For this review, take the finished solid that the model builds, in its own axes (mm). Face numbers are marked on the shaded views. Round coordinates to 2 decimals unless told otherwise and drop trailing zeros. Write each loop counter-clockwise with the first axis right and the second up, starting at its lowest first coordinate (ties: lowest second). Pieces come first, ordered by that corner, then holes. Notation, with made-up numbers: M 12.5,5 L 23.5,5 A24 ccw 23.5,20 Z; hole C 80.5,-13.5 d4. An arc over 180 degrees is marked long. One line per question, with ' | ' between items.
Solid Edge part; units mm, degrees
sketch "Sketch1" plane through (0, 0, 0) normal (0, 0, 1) x (1, 0, 0)
  line L0 (0, -9.2376) -> (8, -4.6188)
  line L1 (8, -4.6188) -> (8, 4.6188)
  line L2 (8, 4.6188) -> (0, 9.2376)
  line L3 (0, 9.2376) -> (-8, 4.6188)
  line L4 (-8, 4.6188) -> (-8, -4.6188)
  line L5 (-8, -4.6188) -> (0, -9.2376)
  circle A0 centre (0, 0) radius 5
extrude "Protrusion1" add sketch "Sketch1" along normal mid plane 8.4
sketch "Sketch2" plane through (0, 0, 0) normal (0, -1, 0) x (1, 0, 0)
  line L0 (8, 4.2) -> (0, 7.1118)
revolve "RevolvedCutout1" cut sketch "Sketch2" angle 360 about axis through (0, 0, 6.3658) along (0, 0, -1) material side at (4.0171, 0, 5.7029)
mirror "Mirror1" about plane through (0, 0, 0) normal (0, 0, 1) of "RevolvedCutout1"
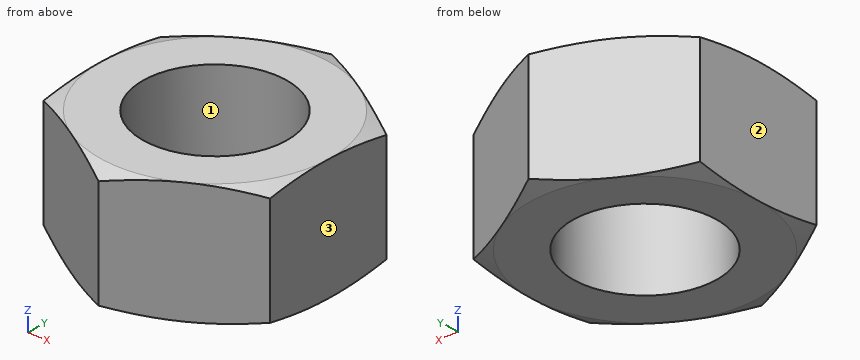
Item 1: To check wall thickness, follow line 1 along Y through (x, z) = (4.25, 3.5); line 2 along Y through (x, z) = (4.5, 3); line 3 along X through (y, z) = (-3.75, -1). State the ranges of each line that lie inside material, in increasing order. Write a range as from..to.
Results:
line 1: -6.78..-2.63, 2.63..6.78 | line 2: -6.64..-2.18, 2.18..6.64 | line 3: -8..-3.31, 3.31..8
Item 2: Insertion check: pin 1 Ø9 at (x, y) = (0, 0) entering from -Z; pin 2 Ø8 at (x, y) = (6, -7.5) entering from -Z; pin 3 Ø2 at (x, z) = (-6, 1.5) entering from +Y; pin 4 Ø1 at (x, z) = (-1, 0.5) entering from +Y. Each pin has a flat end and moves straight along its axis. Give the tip position at first contact, or say it passes through.
Results:
pin 1: through | pin 2: z = -4.2 | pin 3: y = 6.35 | pin 4: y = 8.95
Item 3: Mouldability with a two-part tool opening along X and no side actions: class the marked faces 1, 2 and 3 as +X half, -X half, draft (parallel to the pull), parting line (faces both ways), or undercut.
Results:
face 1: undercut | face 2: -X half | face 3: +X half
Item 4: Take a section at A-A (z = -1.5). Write out the cut boundary in (x, y), then the cut area to 3 significant figures.
Results:
outline: M -8,-4.62 L 0,-9.24 L 8,-4.62 L 8,4.62 L 0,9.24 L -8,4.62 Z; hole C 0,0 d10 | area: 143 mm2
